Can you work these out from the model? Positions are in its coordinate system, mm. A direction names the side the tool comes from. Coordinates: 2 decimals unless noted, no trailing zeros. Loops run counter-clockwise (first coordinate to the right, second up) from the corner with the lowest first, then second, coordinate; pieces in that order, holes last. Notation, with made-up numbers: (-31.75, -28.75) -> (-16.75, -28.75) arc R15 ccw to (-16.75, -15.75) -> close; hole circle Ø3 at (8, -4.75). An arc over 180 degrees is marked (long way). Use one line per item in the form item = value. Start each with the question number.
(1) Imagine slicing it at D-D (x = -72). List the corners of the cut face in (y, z) for me (3 decimals), plus the area to 3 significant figures.
(2) On a 3-axis mill with a long thin cutter (end or side, diameter ignored), from which of +Z, -Z, +X, -X, +Y, -Y can I reach the whole of each face in a straight line? I mean faces 1 (the cylindrical face through (-77.83, -12.88, 0.95)), 2 (the flat face through (-40, -13, 61.595)), 3 (the flat face through (-1, -7.366, 45)). Say none if no direction works.
(3) Imagine slicing it at C-C (z = 12.5). List the corners of the cut face in (x, y) for me (3 decimals).
(4) Thinking about a two-plate mould opening in Y: for faces 4 (the flat face through (-1, -12, 51.584)), 5 (the flat face through (-40, 0, 32)), 6 (the flat face through (-40, -13, 1.905)), which applies, released by +Y, released by -Y, zero draft, split by the parting line, or undercut?
(5) I'm going to push flat-ended pins straight in: pin 1 (1.5 mm diameter, centred on x = -1, y = -12, fed in from -Z); pin 2 (1 mm diameter, centred on x = -18.5, z = 40, fed in from -Y) (3 decimals); pin 3 (1.5 mm diameter, centred on x = -0.5, y = -13, fed in from +Z). Where does each tip first touch, or does it pass through?
(6) I need wall thicknesses on line 1 (X direction, y = -17, z = 50) (3 decimals); line 2 (Z direction, x = -35, y = -9.5) (3 decimals); line 3 (Y direction, x = -36.5, z = 27) (3 decimals). Which ranges of each line are inside material? Lowest first, please. Write a range as [from, to].
(7) Imagine slicing it at A-A (y = -10.75). List the corners of the cut face in (x, z) for me (3 decimals).
(8) Imagine slicing it at B-B (z = 41). List the corners of the cut face in (x, y) for me (3 decimals), plus the area to 3 significant figures.
```python
from build123d import *

# Parameters (mm, degrees)
F0_W     = 78.74
F0_H     = 63.5
F1_DEPTH = 25.4
F2_T     = -1.905
F4_D     = 7.9375
F4_DEPTH = 12.7
F5_W     = 9.525
F5_H     = 12.7
F6_DEPTH = 25.4
F7_R     = 3.175


with BuildPart() as f1:
    # F0 (on Front) → F1 (new body)
    with BuildSketch(Plane.XZ):
        with Locations((-39.37, 31.75)):
            Rectangle(F0_W, F0_H)
    extrude(amount=F1_DEPTH)

    # F2
    f2_openings = [f1.faces().sort_by_distance(p)[0] for p in [
        (-39.37, -25.4, 31.75),
    ]]
    offset(amount=F2_T, openings=f2_openings)

    # F4
    with Locations(Plane.YZ):
        with Locations((-10.64123, 30.9198)):
            Hole(F4_D / 2, depth=F4_DEPTH)

    # F5 (on Right) → F6 (cut)
    with BuildSketch(Plane.YZ):
        with Locations((-12.128341, 45.233511)):
            Rectangle(F5_W, F5_H)
    extrude(amount=-F6_DEPTH, mode=Mode.SUBTRACT)

    # F7
    f7_edges = [f1.edges().sort_by_distance(p)[0] for p in [
        (-78.74, -12.7, 63.5),
        (0, -12.7, 63.5),
        (0, -12.7, 0),
        (-78.74, -12.7, 0),
    ]]
    fillet(f7_edges, radius=F7_R)


solid = f1.part
```
Worked out:
q1.outline = (-25.4, 0) -> (0, 0) -> (0, 63.5) -> (-25.4, 63.5) -> (-25.4, 61.595) -> (-1.905, 61.595) -> (-1.905, 1.905) -> (-25.4, 1.905) -> close
q1.area = 210 mm2
q2.face_1 = -Z, -X, +Y, -Y
q2.face_2 = -Y
q2.face_3 = +X
q3.outline = (-78.74, -25.4) -> (-76.835, -25.4) -> (-76.835, -1.905) -> (-1.905, -1.905) -> (-1.905, -25.4) -> (0, -25.4) -> (0, 0) -> (-78.74, 0) -> close
q4.face_4 = undercut
q4.face_5 = released by +Y
q4.face_6 = zero draft
q5.pin_1 = 0.34
q5.pin_2 = -1.905
q5.pin_3 = 62.85
q6.line_1 = [-78.74, -76.835], [-1.905, 0]
q6.line_2 = [0, 1.905], [61.595, 63.5]
q6.line_3 = [-1.905, 0]
q7.outline = (-78.74, 3.175) arc R3.175 ccw to (-75.565, 0) -> (-3.175, 0) arc R3.175 ccw to (0, 3.175) -> (0, 26.953) -> (-1.905, 26.953) -> (-1.905, 1.905) -> (-76.835, 1.905) -> (-76.835, 61.595) -> (-1.905, 61.595) -> (-1.905, 51.584) -> (0, 51.584) -> (0, 60.325) arc R3.175 ccw to (-3.175, 63.5) -> (-75.565, 63.5) arc R3.175 ccw to (-78.74, 60.325) -> close; (-1.905, 34.887) -> (0, 34.887) -> (0, 38.884) -> (-1.905, 38.884) -> close
q8.outline = (-78.74, -25.4) -> (-76.835, -25.4) -> (-76.835, -1.905) -> (-1.905, -1.905) -> (-1.905, -7.366) -> (0, -7.366) -> (0, 0) -> (-78.74, 0) -> close; (-1.905, -25.4) -> (0, -25.4) -> (0, -16.891) -> (-1.905, -16.891) -> close
q8.area = 221 mm2
